The drawing under review shows one solid part. Ordinate dimensions are in mm from its lowest x, y, z. A direction names the side the tool comes from. Give positions to 0.01 mm unless a question says otherwise; leave off trailing zeros. Loops run counter-clockwise (first coordinate to the right, second up) from the corner with the lowest first, then second, coordinate; pieces in that order, holes last. Notation, with made-up numbers: M 21,14 L 60,14 A4 ccw 60,19 Z; hole C 12.25,76 d7. An arc over 180 degrees is marked long. Put each result on its own line as item: value. Start each with the question number.
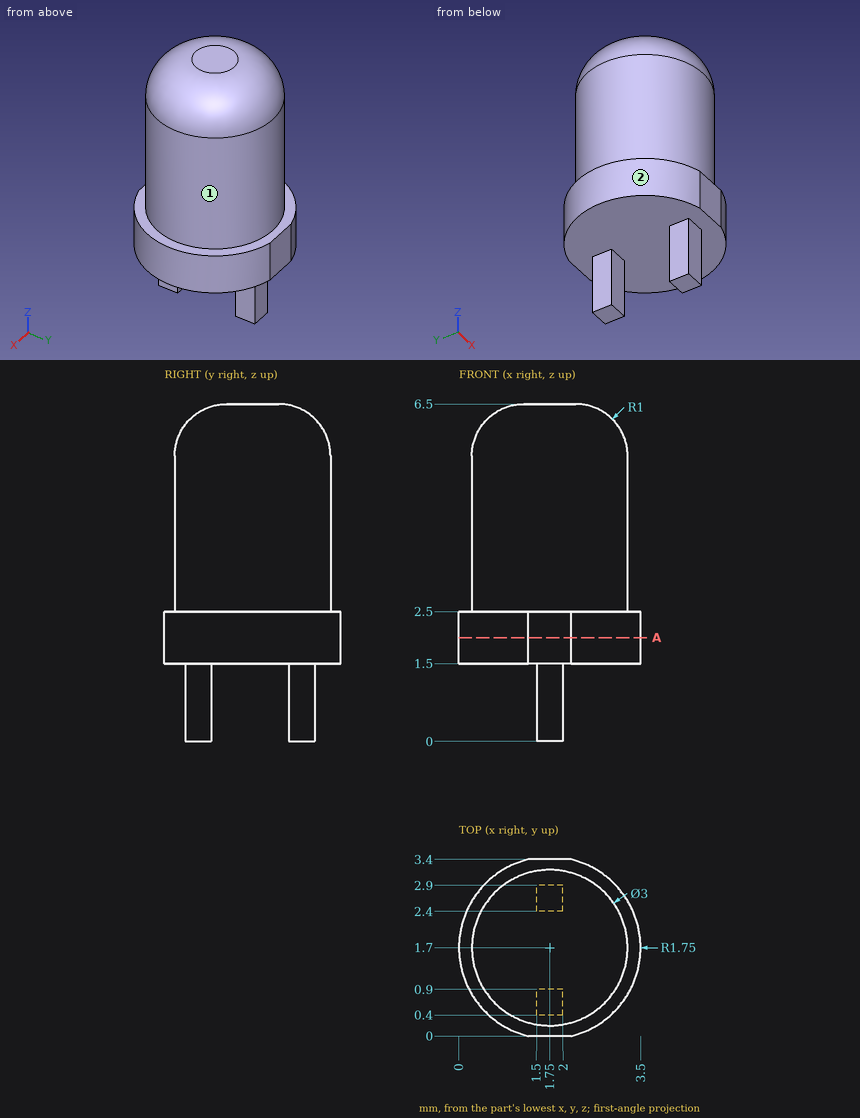
(1) To check wall thickness, follow L1, parallel to Z at x = 2.15, y = 1.6; L2, parallel to Z at x = 0.65, y = 2.95; L3, parallel to Y at x = 0.9, z = 6. State the ranges of each line that lie inside material, in increasing order. Write a range as [from, to].
(2) Insertion check: pin 1 (1 mm diameter, centred on x = 0.5, y = 2, fed in from -Z); pin 2 (1.5 mm diameter, centred on y = 1, z = 3, fed in from -X); pin 3 (0.5 mm diameter, centred on x = 2, z = 1, fed in from -Y). Each pin has a flat end and moves straight along its axis. Give the tip position at first contact, or say it passes through.
(3) For the marked faces 1 and 2, list the 3-axis set-ups (+Z, -Z, +X, -X, +Y, -Y) from which the entire face can be reached by the end or side of a thin tool; tool diameter is ignored.
(4) We need section A-A, the plane z = 2. Write out the cut boundary in (x, y), plus the area to 3 significant figures.
Check sheet entries:
1. L1: z = [1.5, 6.5]
1. L2: z = [1.5, 2.5]
1. L3: y = [0.63, 2.77]
2. pin 1: stops at z = 1.5
2. pin 2: stops at x = 0.01
2. pin 3: stops at y = 0.4
3. face 1: +Z
3. face 2: +Z, -Z, -X
4. outline: M 1.33,0 L 2.17,0 A1.75 ccw 2.17,3.4 L 1.33,3.4 A1.75 ccw Z
4. area: 9.57 mm²
